Answer from the drawing. Dimensions are ordinates in mm from the lowest x, y and z of the part. A direction names the side the tool comes from. Round coordinates to 2 decimals unless told otherwise and drop trailing zeros. Loops run counter-clockwise (first coordinate to the right, second up) from the corner with the lowest first, then second, coordinate; pieces in that order, holes last. Notation, with made-up numbers: (-5.75, 51) -> (49.25, 51) arc R20 ccw to (49.25, 78) -> close; hole circle Ø2 at (17, 42). An arc over 180 degrees is marked (long way). Use CSV: the item, a comma, the result in double quotes. Start each with the question number.
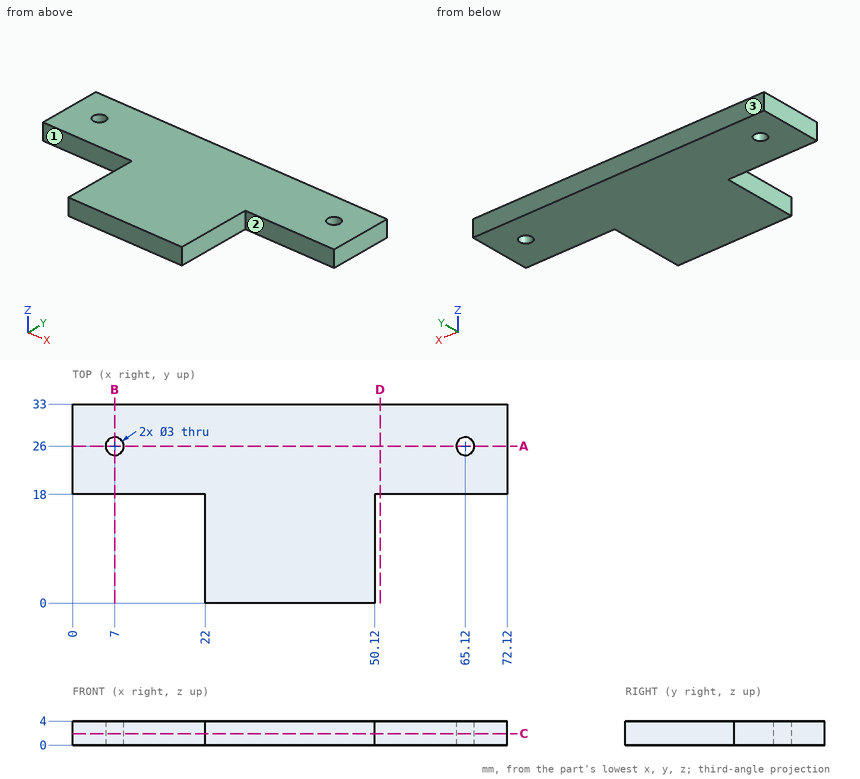
Q1. Section D-D, the plane x = 51 is taken. Write down the section's boundary in (y, z).
Q2. Which of the six approach directions +Z, -Z, +X, -X, +Y, -Y give full straight-line access (tool end or side, diameter ignored) to the marked faces 1, 2 and 3?
Q3. Straight lines are drawn through the part: line 1 (Y direction, x = 7, z = 2.5); line 2 (X direction, y = 25, z = 1.45); line 3 (X direction, y = 11, z = 3.75). For each, find the intervals that lie inside material, in ascending order. Write a range as from..to.
Q4. Section C-C, the plane z = 1.9 is taken. Write down the section's boundary in (x, y).
Q5. Section B-B, the plane x = 7 is taken. Write down the section's boundary in (y, z), and give its area (3 significant figures).
Q6. Section A-A, the plane y = 26 is taken. Write down the section's boundary in (x, z), and give its area (3 significant figures).
Q7. Each of these flat-tipped pins is pushed along its axis until it touches: pin 1 (2 mm diameter, centred on x = 59.5, z = 2.5, fed in from -Y); pin 2 (2.5 mm diameter, centred on x = 65.12, y = 26, fed in from +Z); pin 3 (1.2 mm diameter, centred on y = 13, z = 2, fed in from -X). Where does it stop, or does it pass through?
Report:
1,outline,"(18, 0) -> (33, 0) -> (33, 4) -> (18, 4) -> close"
2,face 1,"+Z, -Z, -X, -Y"
2,face 2,"+Z, -Z, +X, -Y"
2,face 3,"+Z, -Z, +X, -X, +Y"
3,line 1,"y = 18..24.5, 27.5..33"
3,line 2,"x = 0..5.88, 8.12..64, 66.24..72.12"
3,line 3,"x = 22..50.12"
4,outline,"(0, 18) -> (22, 18) -> (22, 0) -> (50.12, 0) -> (50.12, 18) -> (72.12, 18) -> (72.12, 33) -> (0, 33) -> close; hole circle Ø3 at (7, 26); hole circle Ø3 at (65.12, 26)"
5,outline,"(18, 0) -> (24.5, 0) -> (24.5, 4) -> (18, 4) -> close; (27.5, 0) -> (33, 0) -> (33, 4) -> (27.5, 4) -> close"
5,area,"48.0 mm²"
6,outline,"(0, 0) -> (5.5, 0) -> (5.5, 4) -> (0, 4) -> close; (8.5, 0) -> (63.62, 0) -> (63.62, 4) -> (8.5, 4) -> close; (66.62, 0) -> (72.12, 0) -> (72.12, 4) -> (66.62, 4) -> close"
6,area,"264 mm²"
7,pin 1,"stops at y = 18"
7,pin 2,"passes through"
7,pin 3,"stops at x = 22"
